For this review, take the finished solid that the model builds, in its own axes (mm). A direction names the side the tool comes from. Give positions to 0.01 mm unless a question says otherwise; leave off trailing zeros. Loops run counter-clockwise (first coordinate to the right, second up) from the corner with the lowest first, then second, coordinate; pieces in that order, holes last.
```python
from build123d import *

# Parameters (mm, degrees)
F0_W     = 128.136318177
F0_H     = 112.1944747865
F0_R     = 11.9201465669
F1_DEPTH = 147.32
F2_W     = 115.4472436756
F2_H     = 101.3208404183
F3_DEPTH = 112.1954747865
F4_W     = 62.1966458857
F4_H     = 12.2760348022
F5_DEPTH = 32.258
F4_W_2   = 54.5518137515
F4_H_2   = 14.5394429564
F6_DEPTH = 33.02


with BuildPart() as f1:
    # F0 (on Right) → F1 (new body)
    with BuildSketch(Plane.YZ):
        with Locations((-3.1582880765, -0.3007892519)):
            Rectangle(F0_W, F0_H)
        Circle(F0_R, mode=Mode.SUBTRACT)
    extrude(amount=-F1_DEPTH)

    # F2 (on face) → F3 (cut, through all)
    with BuildSketch(Plane.XY.offset(55.7964481413)):
        with Locations((-73.5399918631, -4.2899921536)):
            Rectangle(F2_W, F2_H)
    extrude(amount=-F3_DEPTH, mode=Mode.SUBTRACT)

    # F4 (on face) → F5 (cut)
    with BuildSketch(Plane.XY.offset(55.7964481413)):
        with Locations((-76.4297451824, -61.0884297639)):
            Rectangle(F4_W, F4_H)
    extrude(amount=-F5_DEPTH, mode=Mode.SUBTRACT)

    # F4 (on face) → F6 (cut)
    with BuildSketch(Plane.XY.offset(55.7964481413)):
        with Locations((-86.5978654474, 53.6401495337)):
            Rectangle(F4_W_2, F4_H_2)
    extrude(amount=-F6_DEPTH, mode=Mode.SUBTRACT)


solid = f1.part
```
Item 1: Take a section at D-D on y = -29. Give the boundary of the cut face in (x, z), and give its area (3 significant figures).
Answer:
outline: (-147.32, -56.4) - (-131.26, -56.4) - (-131.26, 55.8) - (-147.32, 55.8) - close; (-15.82, -56.4) - (0, -56.4) - (0, 55.8) - (-15.82, 55.8) - close
area: 3,580 mm2
Item 2: Clearance check with flat-ended pins moving along their axes: pin 1 Ø7.5 at (x, y) = (-96, 52.5) entering from +Z; pin 2 Ø13.5 at (x, y) = (-72.5, -58.5) entering from +Z. State where each tip first meets the part, or that it passes through.
Answer:
pin 1: stops at z = 22.78
pin 2: stops at z = 23.54
Item 3: Tool access review of faces 1 (the cylindrical face through (-7.8, 11.37, 3.58)), 2 (the flat face through (-87, 54, 22.776)), 3 (the flat face through (-74, -54.95, -12)), 4 (the flat face through (-45.331, -61, 40)), 5 (the flat face through (-107.528, -61, 40)): name each direction out of +Z, -Z, +X, -X, +Y, -Y from which nothing blocks a thin tool from reaching the whole face with its end or side.
Answer:
face 1: +X, -X
face 2: +Z, +Y
face 3: +Z, -Z
face 4: +Z, -Y
face 5: +Z, +Y, -Y
Item 4: The part is to be moulded in two halves that separate along Y. For faces 6 (the flat face through (-147.32, -4, 13)), 7 (the flat face through (-73, 60.91, -1)), 8 (the cylindrical face through (-139.18, 11.37, 3.58)), say which applies: released by +Y, released by -Y, zero draft, split by the parting line, or undercut.
Answer:
face 6: zero draft
face 7: released by +Y
face 8: undercut
Item 5: For L1, parallel to X at y = -28, z = 4.5; L2, parallel to Y at x = -94, z = -30.5; L3, parallel to Y at x = -10.5, z = 0.5, list the stretches that pass through material, from the lowest coordinate up.
Answer:
L1: x = -147.32 to -131.26, -15.82 to 0
L2: y = -67.23 to -54.95, 46.37 to 60.91
L3: y = -67.23 to -11.91, 11.91 to 60.91
Item 6: Take a section at A-A on x = -124.5. Give the boundary of the cut face in (y, z).
Answer:
outline: (-67.23, -56.4) - (-54.95, -56.4) - (-54.95, 55.8) - (-67.23, 55.8) - close; (46.37, -56.4) - (60.91, -56.4) - (60.91, 55.8) - (46.37, 55.8) - close
Item 7: Take a section at B-B on y = 0. Give the boundary of the cut face in (x, z), and give its area (3 significant figures).
Answer:
outline: (-147.32, -56.4) - (-131.26, -56.4) - (-131.26, -11.92) - (-147.32, -11.92) - close; (-147.32, 11.92) - (-131.26, 11.92) - (-131.26, 55.8) - (-147.32, 55.8) - close; (-15.82, -56.4) - (0, -56.4) - (0, -11.92) - (-15.82, -11.92) - close; (-15.82, 11.92) - (0, 11.92) - (0, 55.8) - (-15.82, 55.8) - close
area: 2,820 mm2
Item 8: Take a section at C-C on z = 41. Give the boundary of the cut face in (x, y), and give its area (3 significant figures).
Answer:
outline: (-147.32, -67.23) - (-107.53, -67.23) - (-107.53, -54.95) - (-131.26, -54.95) - (-131.26, 46.37) - (-113.87, 46.37) - (-113.87, 60.91) - (-147.32, 60.91) - close; (-59.32, 46.37) - (-15.82, 46.37) - (-15.82, -54.95) - (-45.33, -54.95) - (-45.33, -67.23) - (0, -67.23) - (0, 60.91) - (-59.32, 60.91) - close
area: 5,620 mm2
